Can you work these out from the drawing? Everything is in mm from the part's minimum corner. Coordinates: 2 decimals unless noted, no trailing zeros. Order: outer loops, then holes, each group sorted by start corner. A loop starts at its lowest first (then second) coordinate and runs counter-clockwise, first axis right, second up. Notation, with made-up numbers: (81, -35.5) - (93, -35.5) arc R21 cw to (93, -12.5) - close; hole circle Ø2 at (71.5, 85.25). An arc over 180 degrees is marked (long way). One line per item, written item: value.
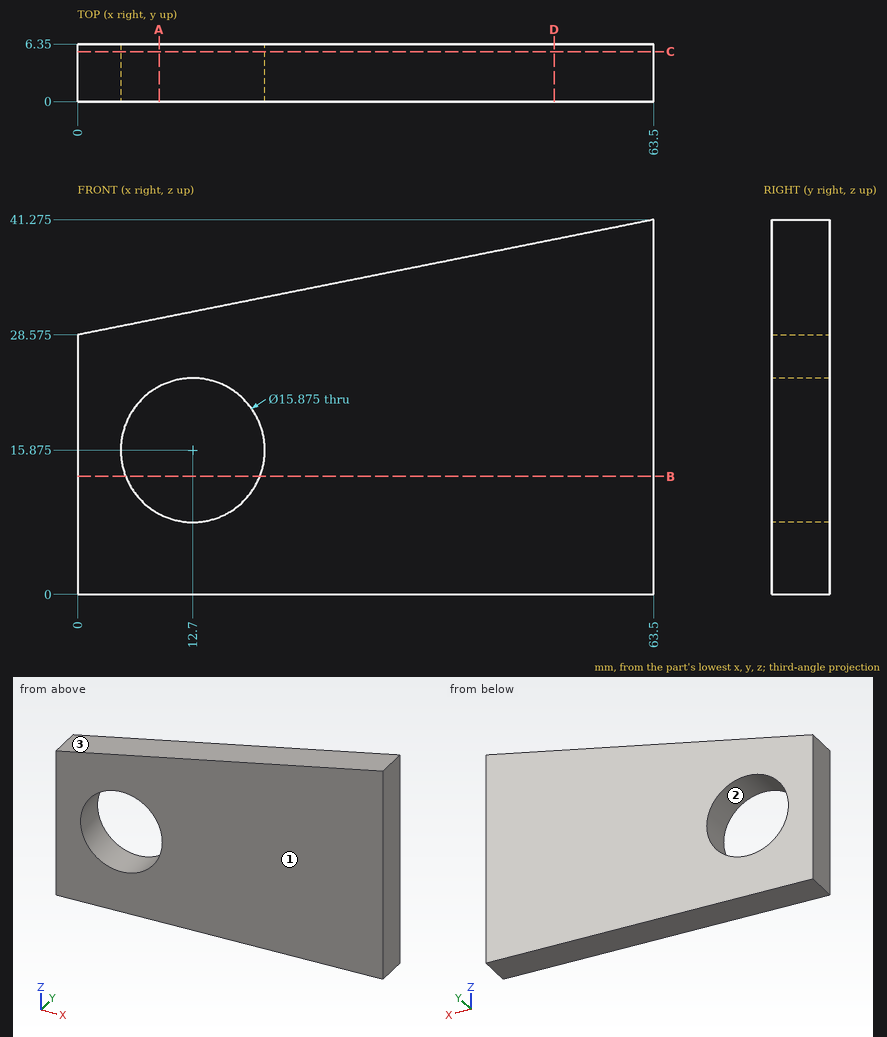
Item 1: Thinking about a two-plate mould opening in Z: for the marked faces 1, 2 and 3, which applies, pulls with the +Z half, pulls with the -Z half, needs draft (parallel to the pull), parting line crosses it, or undercut?
Conclusion:
face 1: needs draft
face 2: undercut
face 3: pulls with the +Z half
Item 2: I want a section at C-C on y = 5.5. Please give me the cut outline in (x, z) (1 decimal), then the cut area to 3 significant figures.
Conclusion:
outline: (0, 0) - (63.5, 0) - (63.5, 41.3) - (0, 28.6) - close; hole circle Ø15.9 at (12.7, 15.9)
area: 2,020 mm²
Item 3: I want a section at B-B on z = 13. Please give me the cut outline in (x, y).
Conclusion:
outline: (0, 0) - (5.3, 0) - (5.3, 6.35) - (0, 6.35) - close; (20.1, 0) - (63.5, 0) - (63.5, 6.35) - (20.1, 6.35) - close
Item 4: I want a section at A-A on x = 9. Please give me the cut outline in (y, z) (3 decimals), then the cut area to 3 significant figures.
Conclusion:
outline: (0, 0) - (6.35, 0) - (6.35, 8.853) - (0, 8.853) - close; (0, 22.897) - (6.35, 22.897) - (6.35, 30.375) - (0, 30.375) - close
area: 104 mm²
Item 5: If I drill on probe 1 along X at (y, z) = (2.5, 9); probe 2 along X at (y, z) = (1, 21.5); probe 3 along Z at (x, y) = (12.7, 4) (1 decimal), over which ranges is the centre line in solid material (lowest first)?
Conclusion:
probe 1: 0 to 8.73, 16.67 to 63.5
probe 2: 0 to 7.1, 18.3 to 63.5
probe 3: 0 to 7.9, 23.8 to 31.1
Item 6: I want a section at D-D on x = 52.5. Please give me the cut outline in (y, z) (3 decimals), then the cut area to 3 significant figures.
Conclusion:
outline: (0, 0) - (6.35, 0) - (6.35, 39.075) - (0, 39.075) - close
area: 248 mm²
